The figure shows three views and two pictorial views of one solid part (mm, origin at its lowest corner). Answer the questions. A direction names the side the tool comes from. Give positions to 0.01 mm unless a question says otherwise; leave off trailing zeros. Order: outer loops, then holes, each group sorted by start corner. A loop starts at its lowest first (then second) coordinate and runs counter-clockwise, first axis right, second up. Notation, with made-up numbers: M 81,64 L 117,64 A19 ccw 117,72 Z; hole C 68.25,12.5 d2. An arc over 180 degrees is marked long. Write item = value, one per line. Start each with the question number.
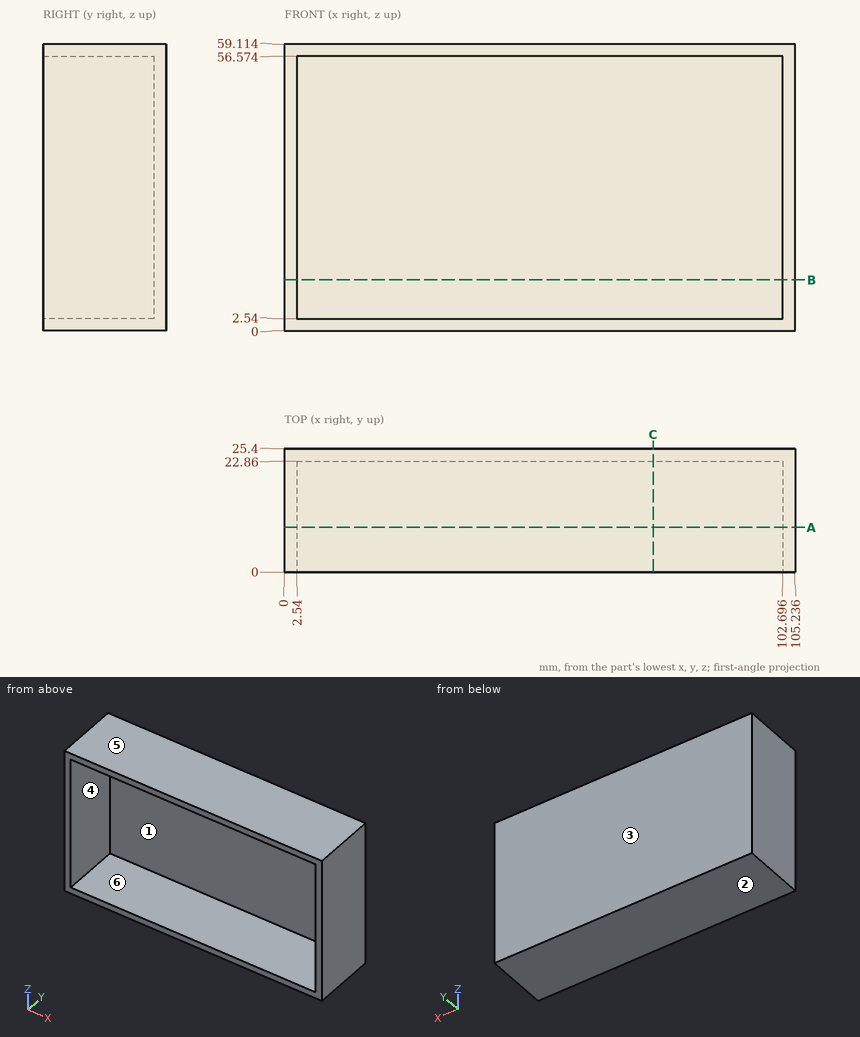
1) Find section C-C on x = 76. Determine the outline of the cut face in (y, z) (1 decimal).
2) Find section B-B on z = 10.5. Determine the outline of the cut face in (x, y).
3) Find section A-A on y = 9.25. Determine the outline of the cut face in (x, z) (1 decimal).
4) For the marked faces 1 and 2, determine the directions among +Z, -Z, +X, -X, +Y, -Y from which every point of the face is accessible in a straight line to the end or side of a thin tool.
5) For a pull along Z with two mould halves and no side action, classify the marked faces 3, 4, 5 and 6 as pulls with the +Z half, pulls with the -Z half, needs draft (parallel to the pull), parting line crosses it, or undercut.
6) This flat-tipped pin is pushed along its axis until it touches: P1, Ø12, axis at x = 51.5, z = 29, coming from the -Y side. Where does it stop, or does it pass through?
7) Find the intervals of material crossed by probe 1 along X at (y, z) = (20.5, 37); probe 2 along Z at (x, y) = (51, 14) (1 decimal); probe 3 along Y at (x, z) = (76.5, 55), in increasing order. Write a range as [from, to].
Numbers:
q1.outline = M 0,0 L 25.4,0 L 25.4,59.1 L 0,59.1 L 0,56.6 L 22.9,56.6 L 22.9,2.5 L 0,2.5 Z
q2.outline = M 0,0 L 2.54,0 L 2.54,22.86 L 102.7,22.86 L 102.7,0 L 105.24,0 L 105.24,25.4 L 0,25.4 Z
q3.outline = M 0,0 L 105.2,0 L 105.2,59.1 L 0,59.1 Z; hole M 2.5,2.5 L 102.7,2.5 L 102.7,56.6 L 2.5,56.6 Z
q4.face_1 = -Y
q4.face_2 = -Z, +X, -X, +Y, -Y
q5.face_3 = needs draft
q5.face_4 = undercut
q5.face_5 = pulls with the +Z half
q5.face_6 = undercut
q6.P1 = 22.86
q7.probe_1 = [0, 2.54], [102.7, 105.24]
q7.probe_2 = [0, 2.5], [56.6, 59.1]
q7.probe_3 = [22.86, 25.4]
